```python
from build123d import *

# Parameters (mm, degrees)
SKETCH1_W           = 23.25
SKETCH1_H           = 42
BOSS_EXTRUDE1_DEPTH = 2
SKETCH2_W           = 23.25
SKETCH2_H           = 42
SKETCH2_W_2         = 19.25
SKETCH2_H_2         = 38
BOSS_EXTRUDE2_DEPTH = 5
SKETCH3_R           = 1.525
SKETCH3_W           = 5
SKETCH3_H           = 2.8
BOSS_EXTRUDE3_DEPTH = 6
SKETCH4_W           = 7.25
SKETCH4_H           = 20.225
SKETCH4_W_2         = 7.988530752
SKETCH4_H_2         = 1.975
BOSS_EXTRUDE4_DEPTH = 4
SKETCH5_W           = 5.2
SKETCH5_H           = 4.5
CUT_EXTRUDE1_DEPTH  = 3
CUT_EXTRUDE3_DEPTH  = 3
CUT_EXTRUDE4_DEPTH  = 3
CUT_EXTRUDE5_DEPTH  = 3
FILLET1_R           = 1


with BuildPart() as part:
    # Sketch1 → Boss-Extrude1 (new body)
    with BuildSketch(Plane.XY):
        Rectangle(SKETCH1_W, SKETCH1_H)
    extrude(amount=BOSS_EXTRUDE1_DEPTH)

    # Sketch2 → Boss-Extrude2 (add)
    with BuildSketch(Plane.XY.offset(2)):
        Rectangle(SKETCH2_W, SKETCH2_H)
        Rectangle(SKETCH2_W_2, SKETCH2_H_2, mode=Mode.SUBTRACT)
    extrude(amount=BOSS_EXTRUDE2_DEPTH)

    # Sketch3 → Boss-Extrude3 (add)
    with BuildSketch(Plane.XY.offset(2)):
        with Locations((0.3, -6.225)):
            Circle(SKETCH3_R)
        with Locations((-7.125, -14.6)):
            Rectangle(SKETCH3_W, SKETCH3_H)
        with Locations((7.125, -14.6)):
            Rectangle(SKETCH3_W, SKETCH3_H)
    extrude(amount=BOSS_EXTRUDE3_DEPTH)

    # Sketch4 → Boss-Extrude4 (add)
    with BuildSketch(Plane.XY.offset(2)):
        with Locations((0, 6.3875)):
            Rectangle(SKETCH4_W, SKETCH4_H)
        with Locations((0.159770615, -9.7125)):
            Rectangle(SKETCH4_W_2, SKETCH4_H_2)
    extrude(amount=BOSS_EXTRUDE4_DEPTH)

    # Sketch5 → Cut-Extrude1 (cut, through all)
    with BuildSketch(Plane.XZ.offset(-19)):
        with Locations((0, 7)):
            Rectangle(SKETCH5_W, SKETCH5_H)
    extrude(amount=-CUT_EXTRUDE1_DEPTH, mode=Mode.SUBTRACT)

    # Sketch6 → Cut-Extrude3 (cut, through all)
    with BuildSketch(Plane(origin=(0, -19, 0), x_dir=(1, 0, 0), z_dir=(0, 1, 0))):
        with BuildLine():
            Line((-2.5, -7), (2.5, -7))
            ThreePointArc((2.5, -7), (0, -4.5), (-2.5, -7))
        make_face()
    extrude(amount=-CUT_EXTRUDE3_DEPTH, mode=Mode.SUBTRACT)

    # Sketch7 → Cut-Extrude4 (cut, through all)
    with BuildSketch(Plane(origin=(-9.625, 0, 0), x_dir=(0, 0, -1), z_dir=(1, 0, 0))):
        Polygon((-2.5, 0), (-2.5, 2.5), (-5, 2.5), (-5, -2.5), (-2.5, -2.5), align=None)
    extrude(amount=-CUT_EXTRUDE4_DEPTH, mode=Mode.SUBTRACT)

    # Sketch8 → Cut-Extrude5 (cut, through all)
    with BuildSketch(Plane.ZY.offset(-9.625)):
        Polygon((2.5, 0), (2.5, -2.5), (5, -2.5), (5, 2.5), (2.5, 2.5), align=None)
    extrude(amount=-CUT_EXTRUDE5_DEPTH, mode=Mode.SUBTRACT)

    # Fillet1
    fillet1_edges = [part.edges().sort_by_distance(p)[0] for p in [
        (0, -21, 0),
        (-11.625, 0, 0),
        (0, 21, 0),
        (11.625, 0, 0),
        (11.625, -21, 3.5),
        (-11.625, -21, 3.5),
        (-11.625, 21, 3.5),
        (11.625, 21, 3.5),
    ]]
    fillet(fillet1_edges, radius=FILLET1_R)


solid = part.part
```
Here's how the part is built. I have some questions about the finished solid (model axes, mm). A direction names the side the tool comes from. Round coordinates to 2 decimals unless told otherwise and drop trailing zeros. Loops run counter-clockwise (first coordinate to the right, second up) from the corner with the lowest first, then second, coordinate; pieces in that order, holes last. Notation, with made-up numbers: (-6, 11) -> (35, 11) arc R17 cw to (35, 16) -> close; hole circle Ø6 at (78.25, 60.25). An arc over 180 degrees is marked (long way). Answer as CSV lines item,"result". Start each with the question number.
1. Imagine slicing it at A-A on y = -1.5. Write out the boundary of the cut face in (x, z) (3 decimals), plus the area to 3 significant figures.
2. Imagine slicing it at C-C on y = 17. Write out the boundary of the cut face in (x, z) (3 decimals).
3. I'm going to push flat-ended pins straight in: P1, Ø1, axis at x = 1.5, y = -10, coming from the +Z side; P2, Ø1, axis at x = 5.5, y = 13.5, coming from the +Z side; P3, Ø1.5, axis at y = 0, z = 3.5, coming from the +X side (3 decimals). Where does each tip first touch, or does it pass through?
4. For faces 5 (the face through (0.149, -20.715, 0.301)), 6 (the face through (0, 20, 4.75)), 7 (the face through (-11, -2.5, 4)), 8 (the face through (1.12, -4.94, 4.96)), 9 (the face through (11, 0, 5)), which set-ups out of +Z, -Z, +X, -X, +Y, -Y let a thin tool reach every point of the face, with its end or its side?
5. Imagine slicing it at B-B on z = 7.5. Write out the boundary of the cut face in (x, y) (3 decimals).
6. If we mould it in two halves opening along X, with no side actions, what happens to faces 1 (the face through (11.324, 0.28, 0.285)), 2 (the face through (10, 0, 7)), 3 (the face through (-9.625, -14.6, 7.5)), 4 (the face through (0, -8.725, 4))? For each: pulls with the +X half, pulls with the -X half, needs draft (parallel to the pull), parting line crosses it, or undercut.
7. Imagine slicing it at D-D on x = -6.75. Write out the boundary of the cut face in (y, z).
8. I need wall thicknesses on probe 1 along Y at (x, z) = (7, 3); probe 2 along X at (y, z) = (14, 2.25) (3 decimals); probe 3 along X at (y, z) = (-7.5, 5.25) (3 decimals). Which ranges of each line are inside material? Lowest first, please. Write a range as from..to.
Solution:
1,outline,"(-11.625, 1) arc R1 ccw to (-10.625, 0) -> (10.625, 0) arc R1 ccw to (11.625, 1) -> (11.625, 2.5) -> (9.625, 2.5) -> (9.625, 2) -> (3.625, 2) -> (3.625, 6) -> (-3.625, 6) -> (-3.625, 2) -> (-9.625, 2) -> (-9.625, 2.5) -> (-11.625, 2.5) -> close; (-11.625, 5) -> (-9.625, 5) -> (-9.625, 7) -> (-11.625, 7) -> close; (9.625, 5) -> (11.625, 5) -> (11.625, 7) -> (9.625, 7) -> close"
1,area,"85.1 mm²"
2,outline,"(-11.625, 1) arc R1 ccw to (-10.625, 0) -> (10.625, 0) arc R1 ccw to (11.625, 1) -> (11.625, 7) -> (9.625, 7) -> (9.625, 2) -> (-9.625, 2) -> (-9.625, 7) -> (-11.625, 7) -> close"
3,P1,"z = 6"
3,P2,"z = 2"
3,P3,"x = 3.625"
4,face 5,"-Z, +X, -X, -Y"
4,face 6,"+Z, +Y"
4,face 7,"-X"
4,face 8,"+Z"
4,face 9,"+X"
5,outline,"(-9.625, -16) -> (-4.625, -16) -> (-4.625, -13.2) -> (-9.625, -13.2) -> close; circle Ø3.05 at (0.3, -6.225); (4.625, -16) -> (9.625, -16) -> (9.625, -13.2) -> (4.625, -13.2) -> close"
6,face 1,"pulls with the +X half"
6,face 2,"needs draft"
6,face 3,"pulls with the -X half"
6,face 4,"undercut"
7,outline,"(-21, 1) arc R1 ccw to (-20, 0) -> (20, 0) arc R1 ccw to (21, 1) -> (21, 7) -> (19, 7) -> (19, 2) -> (-13.2, 2) -> (-13.2, 8) -> (-16, 8) -> (-16, 2) -> (-19, 2) -> (-19, 7) -> (-21, 7) -> close"
8,probe 1,"-21..-19, -16..-13.2, 19..21"
8,probe 2,"-11.625..-9.625, -3.625..3.625, 9.625..11.625"
8,probe 3,"-11.625..-9.625, -0.537..1.137, 9.625..11.625"
